```python
from build123d import *

# Parameters (mm, degrees)
BOSS_EXTRUDE1_DEPTH      = 5
BOSS_EXTRUDE2_DEPTH      = 15
BOSS_EXTRUDE2_DEPTH_BACK = 10
CUT_EXTRUDE1_DEPTH       = 10
FILLET1_R                = 5


with BuildPart() as part:
    # Sketch1 → Boss-Extrude1 (new body)
    with BuildSketch(Plane(origin=(0, 0, 0), x_dir=(1, 0, 0), z_dir=(0, 1, 0))):
        with BuildLine():
            Line((305, 140), (215, 140))
            ThreePointArc((215, 140), (207.928932188, 142.928932188), (205, 150))
            Line((205, 150), (205, 220))
            ThreePointArc((205, 220), (202.071067812, 227.071067812), (195, 230))
            Line((195, 230), (10, 230))
            ThreePointArc((10, 230), (2.928932188, 227.071067812), (0, 220))
            Line((0, 220), (0, 10))
            ThreePointArc((0, 10), (2.928932188, 2.928932188), (10, 0))
            Line((10, 0), (305, 0))
            ThreePointArc((305, 0), (312.071067812, 2.928932188), (315, 10))
            Line((315, 10), (315, 130))
            ThreePointArc((315, 130), (312.071067812, 137.071067812), (305, 140))
        make_face()
    extrude(amount=BOSS_EXTRUDE1_DEPTH)

    # Sketch3 → Boss-Extrude2 (add, two sides)
    with BuildSketch(Plane(origin=(0, 0, 0), x_dir=(1, 0, 0), z_dir=(0, 1, 0))) as boss_extrude2_sk:
        with BuildLine():
            Line((10, 0), (305, 0))
            ThreePointArc((305, 0), (312.071067812, 2.928932188), (315, 10))
            Line((315, 10), (315, 130))
            ThreePointArc((315, 130), (312.071067812, 137.071067812), (305, 140))
            Line((305, 140), (215, 140))
            ThreePointArc((215, 140), (207.928932188, 142.928932188), (205, 150))
            Line((205, 150), (205, 220))
            ThreePointArc((205, 220), (202.071067812, 227.071067812), (195, 230))
            Line((195, 230), (10, 230))
            ThreePointArc((10, 230), (2.928932188, 227.071067812), (0, 220))
            Line((0, 220), (0, 10))
            ThreePointArc((0, 10), (2.928932188, 2.928932188), (10, 0))
        make_face()
        with BuildLine():
            Line((10, 3), (305, 3))
            ThreePointArc((305, 3), (309.949747468, 5.050252532), (312, 10))
            Line((312, 10), (312, 130))
            ThreePointArc((312, 130), (309.949747468, 134.949747468), (305, 137))
            Line((305, 137), (215, 137))
            ThreePointArc((215, 137), (205.807611845, 140.807611845), (202, 150))
            Line((202, 150), (202, 220))
            ThreePointArc((202, 220), (199.949747468, 224.949747468), (195, 227))
            Line((195, 227), (10, 227))
            ThreePointArc((10, 227), (5.050252532, 224.949747468), (3, 220))
            Line((3, 220), (3, 10))
            ThreePointArc((3, 10), (5.050252532, 5.050252532), (10, 3))
        make_face(mode=Mode.SUBTRACT)
    extrude(amount=BOSS_EXTRUDE2_DEPTH)
    extrude(boss_extrude2_sk.sketch, amount=-BOSS_EXTRUDE2_DEPTH_BACK)

    # Sketch4 → Cut-Extrude1 (cut)
    with BuildSketch(Plane(origin=(315, 0, 0), x_dir=(0, 0, -1), z_dir=(1, 0, 0))):
        with BuildLine():
            Line((50, 15), (50, 13))
            ThreePointArc((50, 13), (52.343145751, 7.343145751), (58, 5))
            Line((58, 5), (62, 5))
            ThreePointArc((62, 5), (67.656854249, 7.343145751), (70, 13))
            Line((70, 13), (70, 15))
            Line((70, 15), (50, 15))
        make_face()
    extrude(amount=-CUT_EXTRUDE1_DEPTH, mode=Mode.SUBTRACT)

    # Fillet1
    fillet1_edges = [part.edges().sort_by_distance(p)[0] for p in [
        (157.5, 0, -3),
        (309.949747468, 0, -5.050252532),
        (312, 0, -70),
        (309.949747468, 0, -134.949747468),
        (260, 0, -137),
        (205.807611845, 0, -140.807611845),
        (202, 0, -185),
        (199.949747468, 0, -224.949747468),
        (102.5, 0, -227),
        (5.050252532, 0, -224.949747468),
        (3, 0, -115),
        (5.050252532, 0, -5.050252532),
    ]]
    fillet(fillet1_edges, radius=FILLET1_R)


solid = part.part
```
Verification items for the finished model (mm, model axes). A direction names the side the tool comes from. Give positions to 0.01 mm unless a question says otherwise; leave off trailing zeros. Write each loop counter-clockwise with the first axis right and the second up, starting at its lowest first coordinate (ties: lowest second). Pieces come first, ordered by that corner, then holes. Notation, with made-up numbers: (-3.75, 4.5) - (25.25, 4.5) arc R26 cw to (25.25, 22.5) - close; hole circle Ø7 at (-7.5, 75). An arc over 180 degrees is marked (long way). Put each result on its own line as item: value.
Q1. Set-up check for faces 1 (the face through (261, 10, -137)), 2 (the face through (309.9, -7.5, -5)), 3 (the face through (261, 3, -140)), 4 (the face through (313.521, 7.281, -67.594)): record each of +Z, -Z, +X, -X, +Y, -Y from which the full face is reachable in a straight line by a thin tool's end or side.
Result:
face 1: +Y
face 2: -Y
face 3: -Z, +X, +Y, -Y
face 4: +X, +Y
Q2. Section check A-A on x = 247.5. Record the cut outline in (y, z), and give its area (3 significant figures).
Result:
outline: (-10, -140) - (15, -140) - (15, -137) - (5, -137) - (5, -3) - (15, -3) - (15, 0) - (-10, 0) - (-10, -3) - (-5, -3) arc R5 cw to (0, -8) - (0, -132) arc R5 cw to (-5, -137) - (-10, -137) - close
area: 831 mm2
Q3. Scan lines: probe 1 along Z at (x, y) = (144, -7.25); probe 2 along X at (y, z) = (7.25, -181.5); probe 3 along X at (y, z) = (8.5, -30). Record each from-to range of solid material in increasing order. Write a range as from..to.
Result:
probe 1: -230..-227, -3..0
probe 2: 0..3, 202..205
probe 3: 0..3, 312..315
Q4. Mould release check, pull along Z, two halves, no side actions. Record for faces 5 (the face through (205.909, -7.465, -140.707)), 6 (the face through (205.909, 9.93, -140.707)), 7 (the face through (315, 3, -69)), 8 (the face through (208.01, 2.68, -142.85)): released by +Z, released by -Z, zero draft, split by the parting line, or undercut.
Result:
face 5: undercut
face 6: undercut
face 7: zero draft
face 8: released by -Z
Q5. Section check B-B on z = -204. Record the cut outline in (x, y), and give its area (3 significant figures).
Result:
outline: (0, -10) - (3, -10) - (3, -5) arc R5 cw to (8, 0) - (197, 0) arc R5 cw to (202, -5) - (202, -10) - (205, -10) - (205, 15) - (202, 15) - (202, 5) - (3, 5) - (3, 15) - (0, 15) - close
area: 1,160 mm2
Q6. Depth check by flat-ended pin: P1, Ø1.5, axis at x = 84.5, z = -123, coming from the -Y side; P2, Ø4, axis at x = 218, y = -7, coming from the -Z side; P3, Ø2, axis at x = 314, y = 14.5, coming from the +Z side. Enter the tip coordinate at first touch or a pass-through.
Result:
P1: y = 0
P2: z = -140
P3: z = -4
